```python
from build123d import *

# Parameters (mm, degrees)
BOSS_EXTRUDE1_DEPTH                = 9
F_6_0_6_DIAMETER_HOLE1_AT_2_COUNT  = 2
F_6_0_6_DIAMETER_HOLE1_AT_2_PITCH  = 148.638420336
F_6_0_6_DIAMETER_HOLE1_AT_3_COUNT  = 2
F_6_0_6_DIAMETER_HOLE1_AT_3_PITCH  = 267.921966251
F_6_0_6_DIAMETER_HOLE1_AT_4_COUNT  = 2
F_6_0_6_DIAMETER_HOLE1_AT_4_PITCH  = 267.921966251
F_6_0_6_DIAMETER_HOLE1_AT_5_COUNT  = 2
F_6_0_6_DIAMETER_HOLE1_AT_5_PITCH  = 148.638420336
F_6_0_6_DIAMETER_HOLE1_AT_6_COUNT  = 2
F_6_0_6_DIAMETER_HOLE1_AT_6_PITCH  = 519.685077715
F_6_0_6_DIAMETER_HOLE1_AT_7_COUNT  = 2
F_6_0_6_DIAMETER_HOLE1_AT_7_PITCH  = 519.685077715
F_6_0_6_DIAMETER_HOLE1_AT_8_COUNT  = 2
F_6_0_6_DIAMETER_HOLE1_AT_8_PITCH  = 707.705150469
F_6_0_6_DIAMETER_HOLE1_AT_9_COUNT  = 2
F_6_0_6_DIAMETER_HOLE1_AT_9_PITCH  = 707.705150469
F_6_0_6_DIAMETER_HOLE1_AT_10_COUNT = 2
F_6_0_6_DIAMETER_HOLE1_AT_10_PITCH = 799.1
F_6_0_6_DIAMETER_HOLE3_D           = 6
F_6_0_6_DIAMETER_HOLE3_DEPTH       = 34.5
F_6_0_6_DIAMETER_HOLE3_TIP         = 1.802581857
F_6_0_6_DIAMETER_HOLE4_AT_2_COUNT  = 2
F_6_0_6_DIAMETER_HOLE4_AT_2_PITCH  = 246
F_6_0_6_DIAMETER_HOLE5_AT_2_COUNT  = 2
F_6_0_6_DIAMETER_HOLE5_AT_2_PITCH  = 56
F_6_0_6_DIAMETER_HOLE5_AT_3_COUNT  = 2
F_6_0_6_DIAMETER_HOLE5_AT_3_PITCH  = 164
F_6_0_6_DIAMETER_HOLE5_AT_4_COUNT  = 2
F_6_0_6_DIAMETER_HOLE5_AT_4_PITCH  = 173.297432179


with BuildPart() as part:
    # Sketch1 → Boss-Extrude1 (new body)
    with BuildSketch(Plane(origin=(0, 0, 0), x_dir=(1, 0, 0), z_dir=(0, 1, 0))):
        Polygon((-150, -125), (-150, 125), (-100, 525), (100, 525), (150, 125), (150, -125), (125, -375), (-125, -375), align=None)
    extrude(amount=BOSS_EXTRUDE1_DEPTH)

    # Sketch5 → Ø6.0 (6) Diameter Hole1 (revolve, cut)
    with BuildSketch(Plane(origin=(0, 9, -512.3), x_dir=(0, 0, 1), z_dir=(1, 0, 0))):
        Polygon((0, 0), (0, 9), (6, 9), (3, 6), (3, 0), align=None)
    f_6_0_6_diameter_hole1 = revolve(axis=Axis((0, 15.35, -512.3), (0, -1, 0)), mode=Mode.SUBTRACT)

    # Ø6.0 (6) Diameter Hole1 at 2: Ø6.0 (6) Diameter Hole1 ×2
    with Locations(*[Vector(-0.587331323, 0, 0.809346599) * (i * F_6_0_6_DIAMETER_HOLE1_AT_2_PITCH) for i in range(1, F_6_0_6_DIAMETER_HOLE1_AT_2_COUNT)]):
        add(f_6_0_6_diameter_hole1, mode=Mode.SUBTRACT)

    # Ø6.0 (6) Diameter Hole1 at 3: Ø6.0 (6) Diameter Hole1 ×2
    with Locations(*[Vector(-0.325841144, 0, 0.945424534) * (i * F_6_0_6_DIAMETER_HOLE1_AT_3_PITCH) for i in range(1, F_6_0_6_DIAMETER_HOLE1_AT_3_COUNT)]):
        add(f_6_0_6_diameter_hole1, mode=Mode.SUBTRACT)

    # Ø6.0 (6) Diameter Hole1 at 4: Ø6.0 (6) Diameter Hole1 ×2
    with Locations(*[Vector(0.325841144, 0, 0.945424534) * (i * F_6_0_6_DIAMETER_HOLE1_AT_4_PITCH) for i in range(1, F_6_0_6_DIAMETER_HOLE1_AT_4_COUNT)]):
        add(f_6_0_6_diameter_hole1, mode=Mode.SUBTRACT)

    # Ø6.0 (6) Diameter Hole1 at 5: Ø6.0 (6) Diameter Hole1 ×2
    with Locations(*[Vector(0.587331323, 0, 0.809346599) * (i * F_6_0_6_DIAMETER_HOLE1_AT_5_PITCH) for i in range(1, F_6_0_6_DIAMETER_HOLE1_AT_5_COUNT)]):
        add(f_6_0_6_diameter_hole1, mode=Mode.SUBTRACT)

    # Ø6.0 (6) Diameter Hole1 at 6: Ø6.0 (6) Diameter Hole1 ×2
    with Locations(*[Vector(0.167986351, 0, 0.985789321) * (i * F_6_0_6_DIAMETER_HOLE1_AT_6_PITCH) for i in range(1, F_6_0_6_DIAMETER_HOLE1_AT_6_COUNT)]):
        add(f_6_0_6_diameter_hole1, mode=Mode.SUBTRACT)

    # Ø6.0 (6) Diameter Hole1 at 7: Ø6.0 (6) Diameter Hole1 ×2
    with Locations(*[Vector(-0.167986351, 0, 0.985789321) * (i * F_6_0_6_DIAMETER_HOLE1_AT_7_PITCH) for i in range(1, F_6_0_6_DIAMETER_HOLE1_AT_7_COUNT)]):
        add(f_6_0_6_diameter_hole1, mode=Mode.SUBTRACT)

    # Ø6.0 (6) Diameter Hole1 at 8: Ø6.0 (6) Diameter Hole1 ×2
    with Locations(*[Vector(-0.123356457, 0, 0.992362426) * (i * F_6_0_6_DIAMETER_HOLE1_AT_8_PITCH) for i in range(1, F_6_0_6_DIAMETER_HOLE1_AT_8_COUNT)]):
        add(f_6_0_6_diameter_hole1, mode=Mode.SUBTRACT)

    # Ø6.0 (6) Diameter Hole1 at 9: Ø6.0 (6) Diameter Hole1 ×2
    with Locations(*[Vector(0.123356457, 0, 0.992362426) * (i * F_6_0_6_DIAMETER_HOLE1_AT_9_PITCH) for i in range(1, F_6_0_6_DIAMETER_HOLE1_AT_9_COUNT)]):
        add(f_6_0_6_diameter_hole1, mode=Mode.SUBTRACT)

    # Ø6.0 (6) Diameter Hole1 at 10: Ø6.0 (6) Diameter Hole1 ×2
    with Locations(*[(0, 0, i * F_6_0_6_DIAMETER_HOLE1_AT_10_PITCH) for i in range(1, F_6_0_6_DIAMETER_HOLE1_AT_10_COUNT)]):
        add(f_6_0_6_diameter_hole1, mode=Mode.SUBTRACT)

    # Ø6.0 (6) Diameter Hole3
    with Locations(Plane(origin=(0, 0, -512.3), x_dir=(0, 0, -1), z_dir=(0, -1, 0))):
        with Locations((0, 0), (-120.3, 87.3), (-120.3, -87.3), (-253.3, -87.3), (-253.3, 87.3), (-512.3, 87.3), (-512.3, -87.3), (-702.3, -87.3), (-702.3, 87.3), (-799.1, 0)):
            Hole(F_6_0_6_DIAMETER_HOLE3_D / 2, depth=F_6_0_6_DIAMETER_HOLE3_DEPTH)
            with Locations((0, 0, -(F_6_0_6_DIAMETER_HOLE3_DEPTH + F_6_0_6_DIAMETER_HOLE3_TIP / 2))):  # 118° drill point
                Cone(0, F_6_0_6_DIAMETER_HOLE3_D / 2, F_6_0_6_DIAMETER_HOLE3_TIP, mode=Mode.SUBTRACT)

    # Sketch10 → Ø6.0 (6) Diameter Hole4 (revolve, cut)
    with BuildSketch(Plane(origin=(123, 9, 311), x_dir=(0, 0, 1), z_dir=(1, 0, 0))):
        Polygon((0, 0), (0, 9), (6, 9), (3, 6), (3, 0), align=None)
    f_6_0_6_diameter_hole4 = revolve(axis=Axis((123, 15.35, 311), (0, -1, 0)), mode=Mode.SUBTRACT)

    # Ø6.0 (6) Diameter Hole4 at 2: Ø6.0 (6) Diameter Hole4 ×2
    with Locations(*[(-i * F_6_0_6_DIAMETER_HOLE4_AT_2_PITCH, 0, 0) for i in range(1, F_6_0_6_DIAMETER_HOLE4_AT_2_COUNT)]):
        add(f_6_0_6_diameter_hole4, mode=Mode.SUBTRACT)

    # Sketch12 → Ø6.0 (6) Diameter Hole5 (revolve, cut)
    with BuildSketch(Plane(origin=(-82, 9, 363.75), x_dir=(0, 0, 1), z_dir=(1, 0, 0))):
        Polygon((0, 0), (0, 9), (6, 9), (3, 6), (3, 0), align=None)
    f_6_0_6_diameter_hole5 = revolve(axis=Axis((-82, 15.35, 363.75), (0, -1, 0)), mode=Mode.SUBTRACT)

    # Ø6.0 (6) Diameter Hole5 at 2: Ø6.0 (6) Diameter Hole5 ×2
    with Locations(*[(0, 0, -i * F_6_0_6_DIAMETER_HOLE5_AT_2_PITCH) for i in range(1, F_6_0_6_DIAMETER_HOLE5_AT_2_COUNT)]):
        add(f_6_0_6_diameter_hole5, mode=Mode.SUBTRACT)

    # Ø6.0 (6) Diameter Hole5 at 3: Ø6.0 (6) Diameter Hole5 ×2
    with Locations(*[(i * F_6_0_6_DIAMETER_HOLE5_AT_3_PITCH, 0, 0) for i in range(1, F_6_0_6_DIAMETER_HOLE5_AT_3_COUNT)]):
        add(f_6_0_6_diameter_hole5, mode=Mode.SUBTRACT)

    # Ø6.0 (6) Diameter Hole5 at 4: Ø6.0 (6) Diameter Hole5 ×2
    with Locations(*[Vector(0.946349856, 0, -0.323143853) * (i * F_6_0_6_DIAMETER_HOLE5_AT_4_PITCH) for i in range(1, F_6_0_6_DIAMETER_HOLE5_AT_4_COUNT)]):
        add(f_6_0_6_diameter_hole5, mode=Mode.SUBTRACT)


solid = part.part
```
Source: CAD feature listing. Evaluate the final solid. Frame: model axes, mm. Coordinates: 2 decimals unless noted, no trailing zeros. Write each loop counter-clockwise with the first axis right and the second up, starting at its lowest first coordinate (ties: lowest second). Pieces come first, ordered by that corner, then holes. Notation, with made-up numbers: (67.5, 33) -> (94.5, 33) arc R18 cw to (94.5, 38) -> close; hole circle Ø6 at (70, 41). An arc over 180 degrees is marked (long way). Return JSON: item names as keys, results as strings. Group by question number.
1) Ray query, line 1 along Z through (x, y) = (0, 6.25); line 2 along X through (y, z) = (5.3, 0); line 3 along X through (y, z) = (5.15, -392) (3 decimals). Return the intervals inside material, ascending.
2) Section query C-C, the plane z = -239. Return loops of the section in (x, y), plus the area to 3 significant figures.
3) Section query B-B, the plane z = -433. Return loops of the section in (x, y).
4) Contact query for flat-ended pins moving along their axis: P1, Ø7, axis at x = 82, z = 307.75, coming from the -Y side; P2, Ø5, axis at x = -123, z = 311, coming from the -Y side; P3, Ø8, axis at x = 82, z = 363.75, coming from the -Y side; P4, Ø9.5, axis at x = -87.3, z = 190, coming from the -Y side. Output: stop coordinate, or through.
5) Section query A-A, the plane y = 5.5. State how many separate pieces and enclosed holes the cut face has, plus the area to 3 significant figures.
From the geometry:
{
 "1": {"line 1": "-525 to -515.3, -509.3 to 283.8, 289.8 to 375", "line 2": "-150 to -90.3, -84.3 to 84.3, 90.3 to 150", "line 3": "-116.625 to -90.3, -84.3 to 84.3, 90.3 to 116.625"},
 "2": {"outline": "(-135.75, 0) -> (135.75, 0) -> (135.75, 9) -> (-135.75, 9) -> close", "area": "2,440 mm²"},
 "3": {"outline": "(-111.5, 0) -> (111.5, 0) -> (111.5, 9) -> (-111.5, 9) -> close"},
 "4": {"P1": "y = 2.5", "P2": "through", "P3": "y = 2", "P4": "y = 1.25"},
 "5": {"separate pieces": "1", "enclosed holes": "16", "area": "243,000 mm²"}
}
